Check sheet for the drawn part. Datum: minimum x, y, z corner. Units: mm. A direction names the side the tool comes from. Give positions to 0.01 mm unless a question says otherwise; leave off trailing zeros. Loops run counter-clockwise (first coordinate to the right, second up) from the corner with the lowest first, then second, coordinate; pieces in that order, holes last. Notation, with made-up numbers: (-1.5, 42.5) - (42.5, 42.5) arc R19 cw to (42.5, 48.5) - close; hole circle Ø5 at (50, 27). An arc over 180 degrees is marked (long way). Use one line per item in the form item = value.
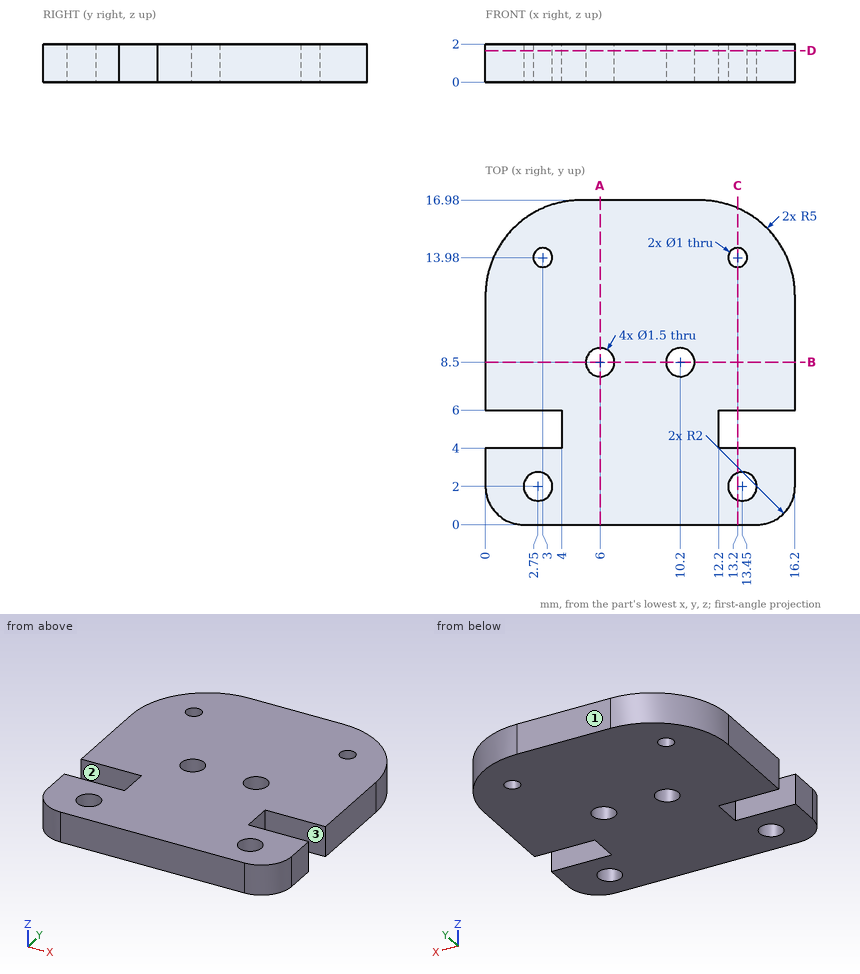
1. Section check B-B, the plane y = 8.5. Record the cut outline in (x, z).
Result set:
outline = (0, 0) - (5.25, 0) - (5.25, 2) - (0, 2) - close; (6.75, 0) - (9.45, 0) - (9.45, 2) - (6.75, 2) - close; (10.95, 0) - (16.2, 0) - (16.2, 2) - (10.95, 2) - close
2. Scan lines: probe 1 along Y at (x, z) = (6, 1.3); probe 2 along Y at (x, z) = (13.5, 1); probe 3 along Y at (x, z) = (1, 0.7). Record each from-to range of solid material in increasing order.
Result set:
probe_1 = 0 to 7.75, 9.25 to 16.98
probe_2 = 0 to 1.25, 2.75 to 4, 6 to 13.58, 14.38 to 16.42
probe_3 = 0.27 to 4, 6 to 14.98
3. Depth check by flat-ended pin: pin 1 Ø0.6 at (y, z) = (5.5, 1) entering from +X; pin 2 Ø0.6 at (x, z) = (2.5, 1.5) entering from +Y. Enter the tip coordinate at first touch or a pass-through.
Result set:
pin_1 = 12.2
pin_2 = 16.47
4. Section check C-C, the plane x = 13.2. Record the cut outline in (y, z).
Result set:
outline = (0, 0) - (1.29, 0) - (1.29, 2) - (0, 2) - close; (2.71, 0) - (4, 0) - (4, 2) - (2.71, 2) - close; (6, 0) - (13.48, 0) - (13.48, 2) - (6, 2) - close; (14.48, 0) - (16.56, 0) - (16.56, 2) - (14.48, 2) - close
5. Section check A-A, the plane x = 6. Record the cut outline in (y, z), then the cut area to 3 significant figures.
Result set:
outline = (0, 0) - (7.75, 0) - (7.75, 2) - (0, 2) - close; (9.25, 0) - (16.98, 0) - (16.98, 2) - (9.25, 2) - close
area = 31.0 mm²
6. Section check D-D, the plane z = 1.65. Record the cut outline in (x, y).
Result set:
outline = (0, 2) arc R2 ccw to (2, 0) - (14.2, 0) arc R2 ccw to (16.2, 2) - (16.2, 4) - (12.2, 4) - (12.2, 6) - (16.2, 6) - (16.2, 11.98) arc R5 ccw to (11.2, 16.98) - (5, 16.98) arc R5 ccw to (0, 11.98) - (0, 6) - (4, 6) - (4, 4) - (0, 4) - close; hole circle Ø1.5 at (2.75, 2); hole circle Ø1 at (3, 13.98); hole circle Ø1.5 at (6, 8.5); hole circle Ø1.5 at (10.2, 8.5); hole circle Ø1.5 at (13.45, 2); hole circle Ø1 at (13.2, 13.98)
7. Tool access check on the marked faces 1, 2 and 3. Record the directions out of +Z, -Z, +X, -X, +Y, -Y that give a thin tool (end or side, any length) a straight path to the whole face; none if there is none.
Result set:
face_1 = +Z, -Z, +X, -X, +Y
face_2 = +Z, -Z, -X
face_3 = +Z, -Z, +X
